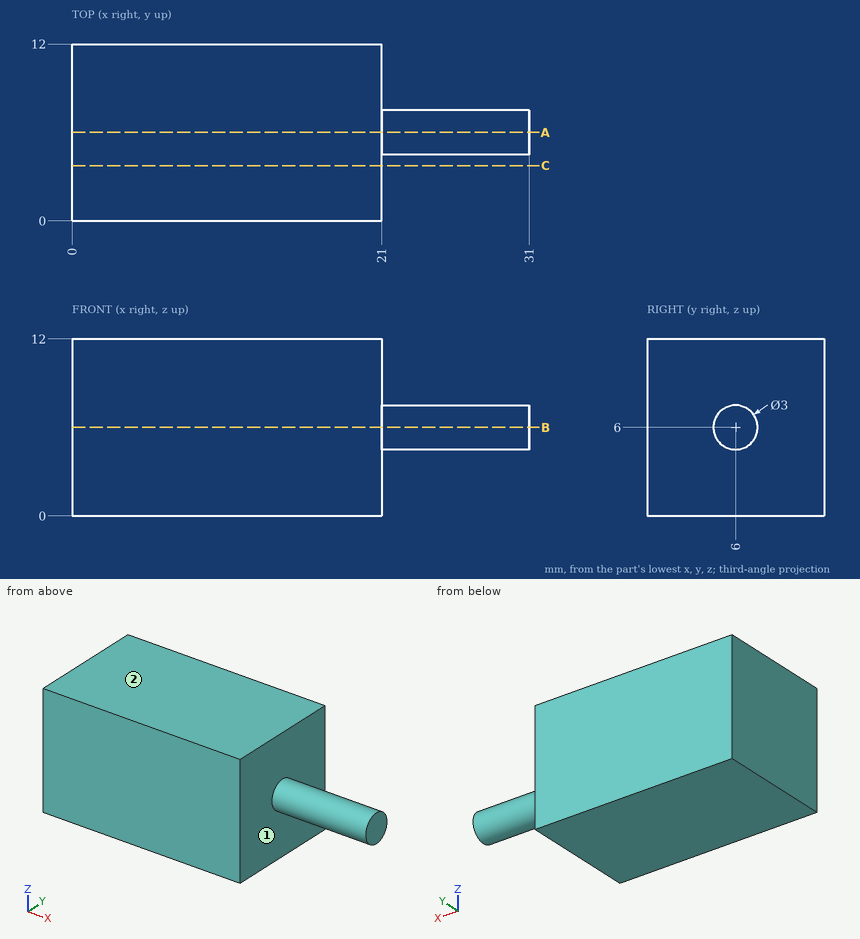
Source: three-view drawing plus pictorial views. Frame: mm from the lowest corner of the part. A direction names the side the tool comes from. Round coordinates to 2 decimals unless told otherwise and drop trailing zeros. Write each loop counter-clockwise with the first axis right and the second up, starting at its lowest first coordinate (ties: lowest second). Pieces come first, ordered by that corner, then holes. Notation, with made-up numbers: M 77,24.25 L 86,24.25 A22 cw 86,43.25 Z; hole C 60,1 d6. An arc over 180 degrees is marked long. Use CSV: the item, a comma, the result in double quotes. Start each with the question number.
Q1. Access query for the marked faces 1 and 2. Directions: +Z, -Z, +X, -X, +Y, -Y. A direction counts if a zero-diameter tool reaches every point of the face in a straight line with its end or side. Return the directions, or none.
Q2. Line query: line 1 (X direction, y = 11.25, z = 7.25); line 2 (Z direction, x = 25, y = 7.25); line 3 (Z direction, x = 29, y = 5). Output: solid intervals per line, ascending. Write a range as from..to.
Q3. Cut plane C-C on y = 3.75. Output: boundary loops of the cut face in (x, z).
Q4. Cut plane A-A on y = 6. Output: boundary loops of the cut face in (x, z).
Q5. First-contact query: P1, Ø2, axis at y = 3.5, z = 2, coming from the +X side; P2, Ø1, axis at x = 25.5, z = 7.5, coming from the +Y side. Flat tips, straight axial feed; report the tip coordinate or a pass-through.
Results found:
1,face 1,"+X"
1,face 2,"+Z, +X, -X, +Y, -Y"
2,line 1,"0..21"
2,line 2,"5.17..6.83"
2,line 3,"4.88..7.12"
3,outline,"M 0,0 L 21,0 L 21,12 L 0,12 Z"
4,outline,"M 0,0 L 21,0 L 21,4.5 L 31,4.5 L 31,7.5 L 21,7.5 L 21,12 L 0,12 Z"
5,P1,"x = 21"
5,P2,"y = 7.12"
